```python
from build123d import *

# Parameters (mm, degrees)
SKETCH1_W             = 42
SKETCH1_H             = 3
BOSS_EXTRUDE1_DEPTH   = 14
BOSS_EXTRUDE1_2_DEPTH = 14
SKETCH2_R             = 1.5
CUT_EXTRUDE1_DEPTH    = 14
SKETCH3_W             = 42
SKETCH3_H             = 11
BOSS_EXTRUDE2_DEPTH   = 5
FILLET1_SIZE          = 3
FILLET1_SIZE_2        = 10


with BuildPart() as part:
    # Sketch1 → Boss-Extrude1 (new body)
    with BuildSketch(Plane(origin=(0, 0, 0), x_dir=(1, 0, 0), z_dir=(0, 1, 0))):
        with Locations((21, -1.5)):
            Rectangle(SKETCH1_W, SKETCH1_H)
    extrude(amount=BOSS_EXTRUDE1_DEPTH)


with BuildPart() as body_2:
    # Sketch1 → Boss-Extrude1 2 (new body)
    with BuildSketch(Plane(origin=(0, 0, 0), x_dir=(1, 0, 0), z_dir=(0, 1, 0))):
        with Locations((21, -9.5)):
            Rectangle(SKETCH1_W, SKETCH1_H)
    extrude(amount=BOSS_EXTRUDE1_2_DEPTH)


with BuildPart() as cut_extrude1_tool:
    # Sketch2 → Cut-Extrude1 (new body)
    with BuildSketch(Plane(origin=(0, 0, 0), x_dir=(-1, 0, 0), z_dir=(0, 0, -1))):
        with BuildLine():
            Line((-36.5, 7), (-35, 7))
            Line((-35, 7), (-33.5, 7))
            ThreePointArc((-33.5, 7), (-35, 8.5), (-36.5, 7))
        make_face()
        with BuildLine():
            Line((-33.5, 7), (-35, 7))
            Line((-35, 7), (-36.5, 7))
            ThreePointArc((-36.5, 7), (-35, 5.5), (-33.5, 7))
        make_face()
        with BuildLine():
            ThreePointArc((-26.5, 7), (-28, 8.5), (-29.5, 7))
            Line((-29.5, 7), (-28, 7))
            Line((-28, 7), (-26.5, 7))
        make_face()
        with BuildLine():
            Line((-28, 7), (-29.5, 7))
            ThreePointArc((-29.5, 7), (-28, 5.5), (-26.5, 7))
            Line((-26.5, 7), (-28, 7))
        make_face()
        with BuildLine():
            ThreePointArc((-5.5, 7), (-7, 8.5), (-8.5, 7))
            Line((-8.5, 7), (-7, 7))
            Line((-7, 7), (-5.5, 7))
        make_face()
        with BuildLine():
            Line((-7, 7), (-8.5, 7))
            ThreePointArc((-8.5, 7), (-7, 5.5), (-5.5, 7))
            Line((-5.5, 7), (-7, 7))
        make_face()
        with Locations((-14, 7)):
            Circle(SKETCH2_R)
    extrude(amount=-CUT_EXTRUDE1_DEPTH)


with BuildPart() as part_1:
    add(part.part)

    # Cut-Extrude1: cut by cut_extrude1_tool
    add(cut_extrude1_tool.part, mode=Mode.SUBTRACT)



with BuildPart() as body_2_1:
    add(body_2.part)

    # Cut-Extrude1: cut by cut_extrude1_tool
    add(cut_extrude1_tool.part, mode=Mode.SUBTRACT)


with BuildPart() as part_2:
    add(part_1.part)

    add(body_2_1.part)  # Boss-Extrude2 merges body 2
    # Sketch3 → Boss-Extrude2 (add)
    with BuildSketch(Plane(origin=(0, 14, 0), x_dir=(1, 0, 0), z_dir=(0, 1, 0))):
        with Locations((21, -5.5)):
            Rectangle(SKETCH3_W, SKETCH3_H)
    extrude(amount=BOSS_EXTRUDE2_DEPTH)

    # Fillet1
    # an asymmetric fillet: 10, 3 mm, written as the material it takes off along each edge
    with BuildSketch(Plane(origin=(67, 19, 0), x_dir=(0, -1, 0), z_dir=(-1, 0, 0))) as fillet1_piece_1:
        with BuildLine():
            Bezier((FILLET1_SIZE, 0), (0, 0), (0, FILLET1_SIZE_2), weights=[1, 0.707106781, 1])
            Line((0, FILLET1_SIZE_2), (0, 0))
            Line((0, 0), (FILLET1_SIZE, 0))
        make_face()
    extrude(amount=92, mode=Mode.SUBTRACT)
    with BuildSketch(Plane(origin=(-25, 19, 11), x_dir=(0, 0, -1), z_dir=(1, 0, 0))) as fillet1_piece_2:
        with BuildLine():
            Bezier((FILLET1_SIZE_2, 0), (0, 0), (0, -FILLET1_SIZE), weights=[1, 0.707106781, 1])
            Line((0, -FILLET1_SIZE), (0, 0))
            Line((0, 0), (FILLET1_SIZE_2, 0))
        make_face()
    extrude(amount=92, mode=Mode.SUBTRACT)


solid = part_2.part
```
Geometry check sheet. Reference: the model listing, model coordinates, mm. A direction names the side the tool comes from. Coordinates: 2 decimals unless noted, no trailing zeros. Order: outer loops, then holes, each group sorted by start corner. A loop starts at its lowest first (then second) coordinate and runs counter-clockwise, first axis right, second up. Notation, with made-up numbers: (18, 23) - (70, 23) arc R33 ccw to (70, 60) - close; hole circle Ø10 at (32, 50.25). An arc over 180 degrees is marked (long way). Answer as a JSON object with one key per item and string values. Group by question number.
Item 1: Scan lines: probe 1 along Z at (x, y) = (11.5, 5); probe 2 along Y at (x, z) = (14, 10.1); probe 3 along Y at (x, z) = (35, 0.95). Record each from-to range of solid material in increasing order.
Item 2: Tool access check on faces 1 (the face through (21, 14, 5)), 2 (the face through (5.8, 7.9, 9.5)). Record the directions out of +Z, -Z, +X, -X, +Y, -Y that give a thin tool (end or side, any length) a straight path to the whole face; none if there is none.
Item 3: Sectioned sample at B-B, the plane x = 7. Give the number of separate pieces and of enclosed holes in the cut face, and give its area (3 significant figures).
Item 4: Draft check along Z on faces 3 (the face through (21, 7, 3)), 4 (the face through (21, 8, 11)), 5 (the face through (0, 9, 9)). Enter one of: +Z half, -Z half, draft (parallel to the pull), parting line (faces both ways), or undercut.
Item 5: Sectioned sample at A-A, the plane y = 9. Record the cut outline in (x, z).
Item 6: Depth check by flat-ended pin: pin 1 Ø2 at (x, z) = (15, 2.5) entering from +Y; pin 2 Ø6 at (y, z) = (13.5, 4) entering from +X; pin 3 Ø1.5 at (x, z) = (20.5, 2.5) entering from +Y; pin 4 Ø2.5 at (x, z) = (16.5, 5.5) entering from -Y. Enter the tip coordinate at first touch or a pass-through.
Resolved:
{
 "1": {"probe 1": "0 to 3, 8 to 11", "probe 2": "0 to 5.5, 8.5 to 17.24", "probe 3": "0 to 5.5, 8.5 to 17.28"},
 "2": {"face 1": "+X, -X, -Y", "face 2": "+Z, -Z"},
 "3": {"separate pieces": "3", "enclosed holes": "0", "area": "109 mm^2"},
 "4": {"face 3": "undercut", "face 4": "+Z half", "face 5": "draft"},
 "5": {"outline": "(0, 0) - (42, 0) - (42, 3) - (0, 3) - close; (0, 8) - (42, 8) - (42, 11) - (0, 11) - close"},
 "6": {"pin 1": "y = 18.28", "pin 2": "x = 42", "pin 3": "y = 18.21", "pin 4": "y = 14"}
}
